Verification items for this drawing (mm, ordinates from the low corner). A direction names the side the tool comes from. Round coordinates to 2 decimals unless told otherwise and drop trailing zeros. Write each loop counter-clockwise with the first axis right and the second up, starting at its lowest first coordinate (ties: lowest second). Pieces come first, ordered by that corner, then holes.
Item 1: Cross-section at A-A (z = 5). Enter the section's corners in (x, y), then the cut area to 3 significant figures.
Item 2: Cross-section at B-B (x = 5). Enter the section's corners in (y, z).
Item 3: Draft check along X on the marked faces 1, 2 and 3. Enter one of: pulls with the +X half, pulls with the -X half, needs draft (parallel to the pull), parting line crosses it, or undercut.
Item 4: Cross-section at D-D (x = 2). Enter the section's corners in (y, z).
Item 5: Depth check by flat-ended pin: P1, Ø1.2, axis at y = 8.5, z = 7, coming from the -X side; P2, Ø2, axis at y = 8, z = 3, coming from the +X side; P3, Ø1.2, axis at y = 9, z = 5, coming from the +X side; P4, Ø5, axis at y = 6.5, z = 2.5, coming from the +X side. Enter the tip coordinate at first touch or a pass-through.
Item 6: Scan lines: probe 1 along Y at (x, z) = (7.7, 5); probe 2 along Y at (x, z) = (3.25, 8.75); probe 3 along X at (y, z) = (6.75, 8). Record each from-to range of solid material in increasing order.
Item 7: Access from +Z, -Z, +X, -X, +Y, -Y to the whole of each face (thin tool, end or side, straight path). Record for the marked faces 4, 5 and 6.
Item 8: Cross-section at C-C (y = 9). Enter the section's corners in (x, z).
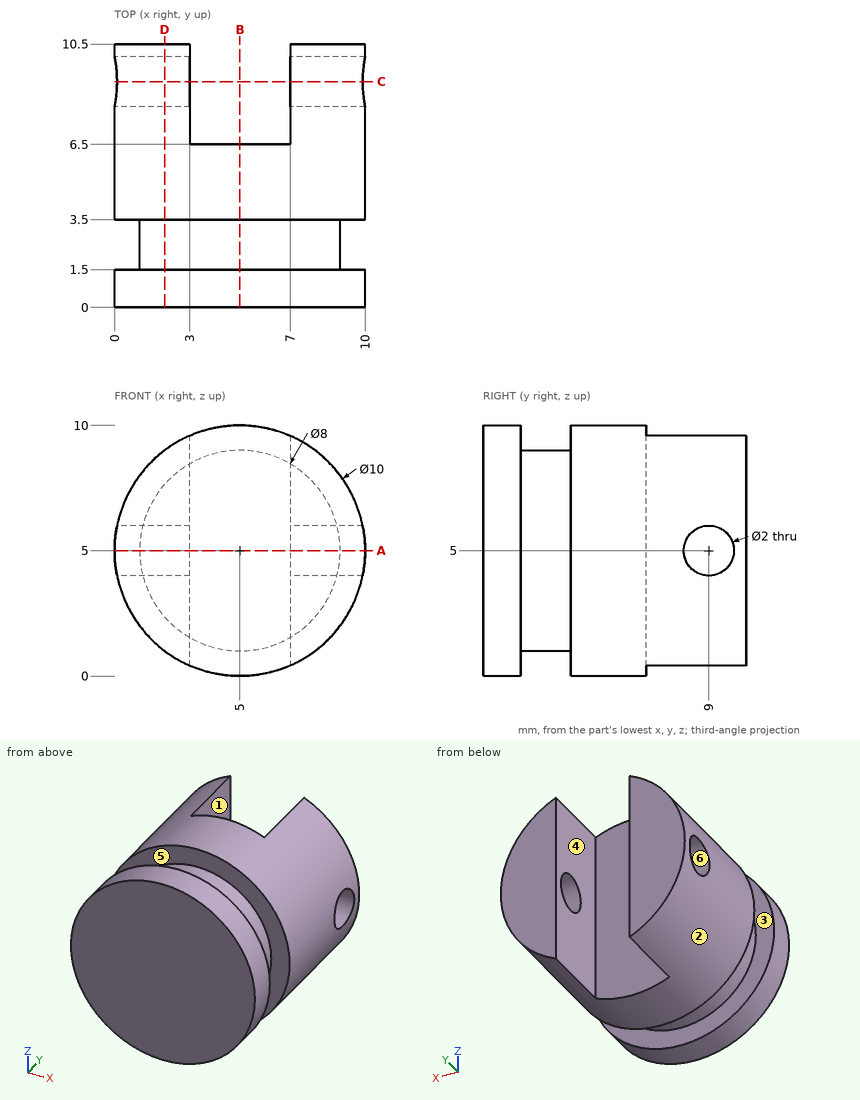
Resolved:
1. outline: (0, 0) - (10, 0) - (10, 1.5) - (9, 1.5) - (9, 3.5) - (10, 3.5) - (10, 8) - (7, 8) - (7, 6.5) - (3, 6.5) - (3, 8) - (0, 8) - (0, 3.5) - (1, 3.5) - (1, 1.5) - (0, 1.5) - close; (0, 10) - (3, 10) - (3, 10.5) - (0, 10.5) - close; (7, 10) - (10, 10) - (10, 10.5) - (7, 10.5) - close
1. area: 73.0 mm2
2. outline: (0, 0) - (1.5, 0) - (1.5, 1) - (3.5, 1) - (3.5, 0) - (6.5, 0) - (6.5, 10) - (3.5, 10) - (3.5, 9) - (1.5, 9) - (1.5, 10) - (0, 10) - close
3. face 1: undercut
3. face 2: parting line crosses it
3. face 3: needs draft
4. outline: (0, 1) - (1.5, 1) - (1.5, 2.35) - (3.5, 2.35) - (3.5, 1) - (10.5, 1) - (10.5, 9) - (3.5, 9) - (3.5, 7.65) - (1.5, 7.65) - (1.5, 9) - (0, 9) - close; hole circle Ø2 at (9, 5)
5. P1: stops at x = 0.2
5. P2: stops at x = 9.9
5. P3: passes through
5. P4: stops at x = 10
6. probe 1: y = 0 to 8, 10 to 10.5
6. probe 2: y = 0 to 1.5, 3.5 to 6.5
6. probe 3: x = 1 to 3, 7 to 9
7. face 4: +Z, -Z, +Y
7. face 5: none
7. face 6: +X, -X
8. outline: (0.1, 4) arc R5 ccw to (3, 0.42) - (3, 4) - close; (0.1, 6) - (3, 6) - (3, 9.58) arc R5 ccw to start; (7, 0.42) arc R5 ccw to (9.9, 4) - (7, 4) - close; (7, 6) - (9.9, 6) arc R5 ccw to (7, 9.58) - close
